Build history of the part. All positions in model axes, mm. A direction names the side the tool comes from. Give positions to 0.01 mm unless a question says otherwise; leave off trailing zeros. Write each loop counter-clockwise with the first axis right and the second up, starting at its lowest first coordinate (ties: lowest second). Pieces come first, ordered by that corner, then holes. Notation, with made-up numbers: M 3,51.5 L 25,51.5 A19 cw 25,86.5 Z; hole C 71.25,17.25 d4. An arc over 180 degrees is marked long. Return JSON: item names as keys, results as strings. Group by question number.
Q1. Band-saw the part on B-B, the plane y = 32.3. Give the cut face in (x, z).
Q2. Band-saw the part on C-C, the plane x = 32.3. Give the cut face in (y, z).
Q3. Flat gauge pins, fed straight in: pin 1 Ø3.5 at (x, z) = (1, 2) entering from -Y; pin 2 Ø1.5 at (x, y) = (-10.5, 21.5) entering from -Z; pin 3 Ø1 at (x, z) = (8, 5) entering from -Y. Where does each tip first touch, or does it go through?
Q4. Tool access for faces 4 (the flat face through (-3.284, 16.596, 13.084)), 5 (the flat face through (0, -13, 1)), 6 (the cylindrical face through (6.042, 6.384, 5.781)): list every direction of +Z, -Z, +X, -X, +Y, -Y with a clear straight run to the whole face (end or side of a thin tool).
Q5. Wall check: probe 1 along Y at (x, z) = (0, 37.4); probe 2 along Z at (x, y) = (20, -23.5); probe 3 along Z at (x, y) = (2, -9.5). Give the ranges that are in metal, low to high.
Q6. Pull direction X, two halves, no side cores. Call faces 1 (the flat face through (15, -15, 35)), 2 (the cylindrical face through (-3.87, 16.55, 20.07)), 3 (the flat face through (-12, -4, 1)): +X half, -X half, draft (parallel to the pull), parting line (faces both ways), or undercut.
Q7. Band-saw the part on A-A, the plane z = 36. Count the separate pieces of the cut face and the enclosed holes in it, then the cut area to 3 significant figures.
from build123d import *

# Parameters (mm, degrees)
SKETCH_1_R               = 35
SKETCH_1_R_2             = 4
EXTRUDE_1_DEPTH          = 40
SKETCH_3_R               = 35
SKETCH_3_R_2             = 19
CUT_EXTRUDE_1_DEPTH      = 35
SKETCH_4_R               = 15
CUT_EXTRUDE_2_DEPTH      = 33.5
SKETCH_6_R               = 1.8
SKETCH_6_R_2             = 2
SKETCH_6_R_3             = 2.2
CUT_EXTRUDE_3_DEPTH      = 41
SKETCH_7_R               = 1.5
SKETCH_7_R_2             = 1.75
CUT_EXTRUDE_4_DEPTH      = 41
CUT_EXTRUDE_5_DEPTH      = 50.497474683
CUT_EXTRUDE_5_DEPTH_BACK = 50.497474683
SKETCH_12_R              = 1.5
SKETCH_12_R_2            = 4
CUT_EXTRUDE_6_DEPTH      = 3


with BuildPart() as part:
    # 草图1 → 凸台-拉伸1 (new body)
    with BuildSketch(Plane.XY):
        Circle(SKETCH_1_R)
        Circle(SKETCH_1_R_2, mode=Mode.SUBTRACT)
    extrude(amount=EXTRUDE_1_DEPTH)

    # 草图3 → 切除-拉伸1 (cut)
    with BuildSketch(Plane.XY):
        Circle(SKETCH_3_R)
        Circle(SKETCH_3_R_2, mode=Mode.SUBTRACT)
    extrude(amount=CUT_EXTRUDE_1_DEPTH, mode=Mode.SUBTRACT)

    # 草图4 → 切除-拉伸2 (cut)
    with BuildSketch(Plane.XY.offset(40)):
        Circle(SKETCH_4_R)
    extrude(amount=-CUT_EXTRUDE_2_DEPTH, mode=Mode.SUBTRACT)

    # 草图6 → 切除-拉伸3 (cut, through all)
    with BuildSketch(Plane.XY):
        with Locations((-24, 0)):
            Circle(SKETCH_6_R)
        with Locations((0, -24)):
            Circle(SKETCH_6_R)
        with Locations((24, 0)):
            Circle(SKETCH_6_R)
        with Locations((0, 24)):
            Circle(SKETCH_6_R)
        with Locations((-32.3, 0)):
            Circle(SKETCH_6_R_2)
        with Locations((32.3, 0)):
            Circle(SKETCH_6_R_3)
        with Locations((0, 32.3)):
            Circle(SKETCH_6_R_2)
        with Locations((0, -32.3)):
            Circle(SKETCH_6_R_2)
    extrude(amount=CUT_EXTRUDE_3_DEPTH, mode=Mode.SUBTRACT)

    # 草图7 → 切除-拉伸4 (cut, through all)
    with BuildSketch(Plane(origin=(0, 0, 0), x_dir=(-1, 0, 0), z_dir=(0, 0, -1))):
        with Locations((-9.5, 0)):
            Circle(SKETCH_7_R)
        with Locations((0, 8)):
            Circle(SKETCH_7_R)
        with Locations((9.5, 0)):
            Circle(SKETCH_7_R)
        with Locations((0, -8)):
            Circle(SKETCH_7_R)
        with Locations((-8.131727984, -8.131727984)):
            Circle(SKETCH_7_R_2)
        with Locations((-8.131727984, 8.131727984)):
            Circle(SKETCH_7_R_2)
        with Locations((8.131727984, 8.131727984)):
            Circle(SKETCH_7_R_2)
        with Locations((8.131727984, -8.131727984)):
            Circle(SKETCH_7_R_2)
    extrude(amount=-CUT_EXTRUDE_4_DEPTH, mode=Mode.SUBTRACT)

    # 草图9 → 切除-拉伸5 (cut, two sides)
    with BuildSketch(Plane(origin=(0, 0, 0), x_dir=(0.707106781, 0.707106781, 0), z_dir=(0.707106781, -0.707106781, 0))) as cut_extrude_5_sk:
        with BuildLine():
            Line((-7.91330988, 20.5), (7.91330988, 20.5))
            ThreePointArc((7.91330988, 20.5), (8.973970052, 20.060660172), (9.41330988, 19))
            Line((9.41330988, 19), (9.41330988, 7))
            ThreePointArc((9.41330988, 7), (8.973970052, 5.939339828), (7.91330988, 5.5))
            Line((7.91330988, 5.5), (-7.91330988, 5.5))
            ThreePointArc((-7.91330988, 5.5), (-8.973970052, 5.939339828), (-9.41330988, 7))
            Line((-9.41330988, 7), (-9.41330988, 19))
            ThreePointArc((-9.41330988, 19), (-8.973970052, 20.060660172), (-7.91330988, 20.5))
        make_face()
    extrude(amount=CUT_EXTRUDE_5_DEPTH, mode=Mode.SUBTRACT)
    extrude(cut_extrude_5_sk.sketch, amount=-CUT_EXTRUDE_5_DEPTH_BACK, mode=Mode.SUBTRACT)

    # 草图12 → 切除-拉伸6 (cut)
    with BuildSketch(Plane(origin=(0, 0, 0), x_dir=(-1, 0, 0), z_dir=(0, 0, -1))):
        with BuildLine():
            ThreePointArc((10, -4), (5.757359313, -5.757359313), (4, -10))
            Line((4, -10), (4, -13))
            Line((4, -13), (0, -13))
            Line((0, -13), (-4, -13))
            Line((-4, -13), (-4, -10))
            ThreePointArc((-4, -10), (-5.757359313, -5.757359313), (-10, -4))
            Line((-10, -4), (-13, -4))
            Line((-13, -4), (-13, 0))
            Line((-13, 0), (-13, 4))
            Line((-13, 4), (-10, 4))
            ThreePointArc((-10, 4), (-5.757359313, 5.757359313), (-4, 10))
            Line((-4, 10), (-4, 13))
            Line((-4, 13), (0, 13))
            Line((0, 13), (4, 13))
            Line((4, 13), (4, 10))
            ThreePointArc((4, 10), (5.757359313, 5.757359313), (10, 4))
            Line((10, 4), (13, 4))
            Line((13, 4), (13, 0))
            Line((13, 0), (13, -4))
            Line((13, -4), (10, -4))
        make_face()
        with Locations((9.5, 0)):
            Circle(SKETCH_12_R, mode=Mode.SUBTRACT)
        with Locations((-9.5, 0)):
            Circle(SKETCH_12_R, mode=Mode.SUBTRACT)
        Circle(SKETCH_12_R_2, mode=Mode.SUBTRACT)
        with Locations((0, -8)):
            Circle(SKETCH_12_R, mode=Mode.SUBTRACT)
        with Locations((0, 8)):
            Circle(SKETCH_12_R, mode=Mode.SUBTRACT)
    extrude(amount=-CUT_EXTRUDE_6_DEPTH, mode=Mode.SUBTRACT)


solid = part.part
From the geometry:
{
 "1": {"outline": "M -13.48,35 L -2,35 L -2,40 L -13.48,40 Z; M 2,35 L 13.48,35 L 13.48,40 L 2,40 Z"},
 "2": {"outline": "M -13.48,35 L -2.2,35 L -2.2,40 L -13.48,40 Z; M 2.2,35 L 13.48,35 L 13.48,40 L 2.2,40 Z"},
 "3": {"pin 1": "stops at y = -19", "pin 2": "stops at z = 35", "pin 3": "stops at y = -17.46"},
 "4": {"face 4": "-X", "face 5": "-Z", "face 6": "none"},
 "5": {"probe 1": "y = -35 to -34.3, -30.3 to -25.8, -22.2 to -15, 15 to 22.2, 25.8 to 30.3, 34.3 to 35", "probe 2": "z = 35 to 40", "probe 3": "z = 3 to 5.5"},
 "6": {"face 1": "draft", "face 2": "-X half", "face 3": "undercut"},
 "7": {"separate pieces": "1", "enclosed holes": "9", "area": "3,050 mm^2"}
}
